```python
from build123d import *

# Parameters (mm, degrees)
F1_DEPTH  = 5
F4_D      = 5.5
F4_DEPTH  = 10
F4_TIP    = 1.6523667023
F5_D      = 5.5
F5_DEPTH  = 10
F5_TIP    = 1.6523667023
F7_D      = 5.5
F7_DEPTH  = 10
F7_TIP    = 1.6523667023
F9_DEPTH  = 6
F11_DEPTH = 6
F12_SIZE  = 5.08
F13_SIZE  = 5.08


with BuildPart() as f1:
    # F0 (on Front) → F1 (new body, symmetric)
    with BuildSketch(Plane.XZ):
        with BuildLine():
            Line((-71.2879747152, 42.1321982205), (-71.2879747152, 28.2593462616))
            Line((-71.2879747152, 28.2593462616), (-22.9098405689, 28.2593462616))
            Line((-22.9098405689, 28.2593462616), (-22.9098405689, 51.0221982205))
            Line((-22.9098405689, 51.0221982205), (-62.3979747152, 51.0221982205))
            ThreePointArc((-62.3979747152, 51.0221982205), (-68.684154, 48.4183775052), (-71.2879747152, 42.1321982205))
        make_face()
        Polygon((-22.9098405689, 28.2593462616), (-71.2879747152, 28.2593462616), (-71.2879747152, -32.6785035431), (69.0129896845, -32.6785035431), (69.0129896845, 28.2593462616), (23.607602343, 28.2593462616), align=None)
        with BuildLine():
            Line((23.607602343, 51.0221982205), (23.607602343, 28.2593462616))
            Line((23.607602343, 28.2593462616), (69.0129896845, 28.2593462616))
            Line((69.0129896845, 28.2593462616), (69.0129896845, 42.1321982205))
            ThreePointArc((69.0129896845, 42.1321982205), (66.4091689693, 48.4183775052), (60.1229896845, 51.0221982205))
            Line((60.1229896845, 51.0221982205), (23.607602343, 51.0221982205))
        make_face()
    extrude(amount=F1_DEPTH, both=True)

    # F4
    with Locations(Plane.XY.offset(51.0221982205)):
        with Locations((-42.6539076421, 0)):
            Hole(F4_D / 2, depth=F4_DEPTH)
            with Locations((0, 0, -(F4_DEPTH + F4_TIP / 2))):  # 118° drill point
                Cone(0, F4_D / 2, F4_TIP, mode=Mode.SUBTRACT)

    # F5
    with Locations(Plane.XY.offset(51.0221982205)):
        with Locations((43.3775149286, 0)):
            Hole(F5_D / 2, depth=F5_DEPTH)
            with Locations((0, 0, -(F5_DEPTH + F5_TIP / 2))):  # 118° drill point
                Cone(0, F5_D / 2, F5_TIP, mode=Mode.SUBTRACT)

    # F7
    with Locations(Plane.XY.offset(28.2593462616)):
        with Locations((0, 0)):
            Hole(F7_D / 2, depth=F7_DEPTH)
            with Locations((0, 0, -(F7_DEPTH + F7_TIP / 2))):  # 118° drill point
                Cone(0, F7_D / 2, F7_TIP, mode=Mode.SUBTRACT)

    # F8 (on face) → F9 (cut)
    with BuildSketch(Plane.XZ.offset(5)):
        with BuildLine():
            Line((-28.2593462616, 25.0004206035), (-28.2593462616, 20.1726239209))
            ThreePointArc((-28.2593462616, 20.1726239209), (-44.6016580305, 41.9345797557), (-65.9063084503, 25.0004206035))
            Line((-65.9063084503, 25.0004206035), (-28.2593462616, 25.0004206035))
        make_face()
        Polygon((-28.2593462616, -32.6785035431), (-28.2593462616, 20.1726239209), (-28.2593462616, 25.0004206035), (-65.9063084503, 25.0004206035), (-65.9063084503, 21.2075540823), (-65.9063084503, -32.6785035431), (-61.2867288291, -32.6785035431), (-61.2867288291, 11.5130664781), (-31.9807417691, 11.5130664781), (-31.9807417691, -32.6785035431), align=None)
    extrude(amount=-F9_DEPTH, mode=Mode.SUBTRACT)

    # F10 (on face) → F11 (cut)
    with BuildSketch(Plane.XZ.offset(5)):
        with BuildLine():
            Line((26.4657004472, 25.0048964569), (63.6281896845, 25.0048964569))
            ThreePointArc((63.6281896845, 25.0048964569), (45.0469450659, 41.3656967057), (26.4657004472, 25.0048964569))
        make_face()
        Polygon((63.6281896845, -32.6785035431), (63.6281896845, 25.0048964569), (26.4657004472, 25.0048964569), (26.4657004472, 20.2626549029), (26.4657004472, -32.6785035431), (31.1232465006, -32.6785035431), (31.1232465006, 11.9440579109), (60.4292335607, 11.9440579109), (60.4292335607, -32.6785035431), align=None)
    extrude(amount=-F11_DEPTH, mode=Mode.SUBTRACT)

    # F12
    f12_edges = [f1.edges().sort_by_distance(p)[0] for p in [
        (-22.909841, 0, 51.022198),
    ]]
    chamfer(f12_edges, length=F12_SIZE)

    # F13
    f13_edges = [f1.edges().sort_by_distance(p)[0] for p in [
        (23.607602, 0, 51.022198),
    ]]
    chamfer(f13_edges, length=F13_SIZE)


solid = f1.part
```
Can you work these out from the model? Positions are in its coordinate system, mm. A direction names the side the tool comes from. Round coordinates to 2 decimals unless told otherwise and drop trailing zeros. Loops run counter-clockwise (first coordinate to the right, second up) from the corner with the lowest first, then second, coordinate; pieces in that order, holes last. Notation, with made-up numbers: (15.25, 0) -> (56.25, 0) arc R14 cw to (56.25, 15) -> close; hole circle Ø2 at (63, 17.25). An arc over 180 degrees is marked (long way). Answer in a Markdown table with one row per item.
Item 1: We'd pull the mould along Y, two halves only. Please class faces 1 (the flat face through (31.123, -2, -11)), 2 (the flat face through (46, -5, -10)), 3 (the cylindrical face through (-39.907, 0.121, 45.952)): released by +Y, released by -Y, zero draft, split by the parting line, or undercut.
Answer block:
| item | result |
|---|---|
| face 1 | zero draft |
| face 2 | released by -Y |
| face 3 | undercut |
Item 2: Suppose I cut it at A-A, the plane z = 34. List the corners of the cut face in (x, y) for me.
Answer block:
| item | result |
|---|---|
| outline | (-71.29, -5) -> (-62.56, -5) -> (-62.56, 1) -> (-31.47, 1) -> (-31.47, -5) -> (-22.91, -5) -> (-22.91, 5) -> (-71.29, 5) -> close; (23.61, -5) -> (30.16, -5) -> (30.16, 1) -> (59.94, 1) -> (59.94, -5) -> (69.01, -5) -> (69.01, 5) -> (23.61, 5) -> close |
Item 3: Suppose I cut it at D-D, the plane x = 11. List the corners of the cut face in (y, z) for me, plus the area to 3 significant figures.
Answer block:
| item | result |
|---|---|
| outline | (-5, -32.68) -> (5, -32.68) -> (5, 28.26) -> (-5, 28.26) -> close |
| area | 609 mm² |
Item 4: If I drill on probe 1 along X at (y, z) = (0.5, -26.5); probe 2 along Y at (x, z) = (0, 22.5); probe 3 along X at (y, z) = (0, 45.75), over which ranges is the centre line in solid material (lowest first)?
Answer block:
| item | result |
|---|---|
| probe 1 | -71.29 to -65.91, -61.29 to -31.98, -28.26 to 26.47, 31.12 to 60.43, 63.63 to 69.01 |
| probe 2 | -5 to -2.75, 2.75 to 5 |
| probe 3 | -70.52 to -45.4, -39.9 to -22.91, 23.61 to 40.63, 46.13 to 68.24 |
Item 5: Suppose I cut it at B-B, the plane x = 38. List the corners of the cut face in (y, z) for me, plus the area to 3 significant figures.
Answer block:
| item | result |
|---|---|
| outline | (-5, -32.68) -> (5, -32.68) -> (5, 51.02) -> (-5, 51.02) -> (-5, 39.99) -> (1, 39.99) -> (1, 11.94) -> (-5, 11.94) -> close |
| area | 669 mm² |
Item 6: Will this pin go through, and if not, where does the flat tip stop? P1, Ø3.5, axis at x = -42.65, y = 0, coming from the +Z side.
Answer block:
| item | result |
|---|---|
| P1 | z = 40.42 |
Item 7: Suppose I cut it at C-C, the plane x = 55.5. List the corners of the cut face in (y, z) for me.
Answer block:
| item | result |
|---|---|
| outline | (-5, -32.68) -> (5, -32.68) -> (5, 51.02) -> (-5, 51.02) -> (-5, 38.18) -> (1, 38.18) -> (1, 11.94) -> (-5, 11.94) -> close |
Item 8: On a 3-axis mill with a long thin cutter (end or side, diameter ignored), from which of +Z, -Z, +X, -X, +Y, -Y can I reach the whole of each face in a straight line? I mean faces 4 (the cylindrical face through (40.755, 0.826, 45.952)), 5 (the flat face through (23.608, 0, 37)), 6 (the cylindrical face through (-44.181, -2.709, 41.876)), 7 (the flat face through (-28.259, -2, -7)). Say none if no direction works.
Answer block:
| item | result |
|---|---|
| face 4 | +Z |
| face 5 | +Z, +Y, -Y |
| face 6 | -Y |
| face 7 | -Z, -Y |
